Could you check a few things on this model? Use its own coordinates, in mm. Face numbers are marked on the shaded views. Give positions to 0.01 mm unless a question says otherwise; leave off trailing zeros. Write each loop counter-clockwise with the first axis right and the second up, starting at its lowest first coordinate (ties: lowest second). Pieces come first, ordered by that corner, then holes. Notation, with made-up numbers: (38.5, 61.25) - (83.5, 61.25) arc R17 ccw to (83.5, 78.25) - close; hole circle Ø6 at (53.25, -20). An arc over 180 degrees is marked (long way). Write item = value, one per line.
from build123d import *

# Parameters (mm, degrees)
SKETCH1_R           = 30
SKETCH1_R_2         = 5
BOSS_EXTRUDE1_DEPTH = 15
FILLET1_R           = 15


with BuildPart() as part:
    # Sketch1 → Boss-Extrude1 (new, symmetric)
    with BuildSketch(Plane(origin=(0, 0, 0), x_dir=(1, 0, 0), z_dir=(0, 1, 0))):
        with BuildLine():
            Line((13.821869985, 37.536061462), (7.39103626, 53.061467459))
            ThreePointArc((7.39103626, 53.061467459), (0, 58), (-7.39103626, 53.061467459))
            Line((-7.39103626, 53.061467459), (-13.821869985, 37.536061462))
            ThreePointArc((-13.821869985, 37.536061462), (-28.284271247, 28.284271247), (-37.536061462, 13.821869985))
            Line((-37.536061462, 13.821869985), (-53.061467459, 7.39103626))
            ThreePointArc((-53.061467459, 7.39103626), (-58, 0), (-53.061467459, -7.39103626))
            Line((-53.061467459, -7.39103626), (-37.536061462, -13.821869985))
            ThreePointArc((-37.536061462, -13.821869985), (-28.284271247, -28.284271247), (-13.821869985, -37.536061462))
            Line((-13.821869985, -37.536061462), (-7.39103626, -53.061467459))
            ThreePointArc((-7.39103626, -53.061467459), (0, -58), (7.39103626, -53.061467459))
            Line((7.39103626, -53.061467459), (13.821869985, -37.536061462))
            ThreePointArc((13.821869985, -37.536061462), (28.284271247, -28.284271247), (37.536061462, -13.821869985))
            Line((37.536061462, -13.821869985), (53.061467459, -7.39103626))
            ThreePointArc((53.061467459, -7.39103626), (58, 0), (53.061467459, 7.39103626))
            Line((53.061467459, 7.39103626), (37.536061462, 13.821869985))
            ThreePointArc((37.536061462, 13.821869985), (28.284271247, 28.284271247), (13.821869985, 37.536061462))
        make_face()
        with Locations(Location((0, 0, 0), (0, 0, 270))):
            Circle(SKETCH1_R, mode=Mode.SUBTRACT)
        with Locations(Location((0, 50, 0), (0, 0, 270))):
            Circle(SKETCH1_R_2, mode=Mode.SUBTRACT)
        with Locations(Location((-50, 0, 0), (0, 0, 270))):
            Circle(SKETCH1_R_2, mode=Mode.SUBTRACT)
        with Locations(Location((50, 0, 0), (0, 0, 270))):
            Circle(SKETCH1_R_2, mode=Mode.SUBTRACT)
        with Locations(Location((0, -50, 0), (0, 0, 270))):
            Circle(SKETCH1_R_2, mode=Mode.SUBTRACT)
    extrude(amount=BOSS_EXTRUDE1_DEPTH, both=True)

    # Fillet1
    fillet1_edges = [part.edges().sort_by_distance(p)[0] for p in [
        (-37.536061462, 0, -13.821869985),
        (-13.821869985, 0, -37.536061462),
        (13.821869985, 0, -37.536061462),
        (37.536061462, 0, -13.821869985),
        (37.536061462, 0, 13.821869985),
        (13.821869985, 0, 37.536061462),
        (-13.821869985, 0, 37.536061462),
        (-37.536061462, 0, 13.821869985),
    ]]
    fillet(fillet1_edges, radius=FILLET1_R)


solid = part.part
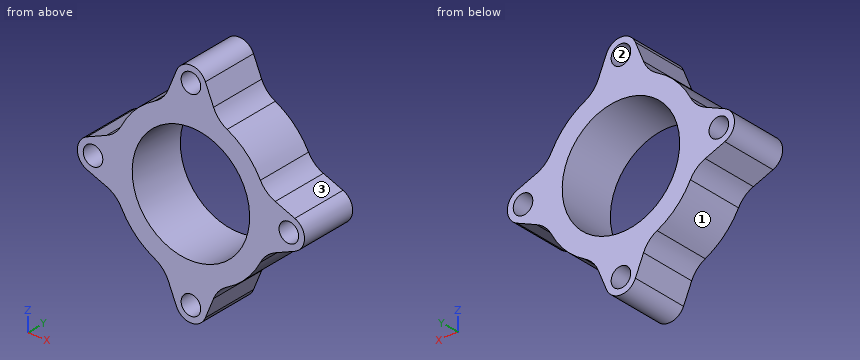
1. If we section it at C-C, the plane y = 2.25: Count the separate pieces of the cut face and the enclosed holes in it, and give its area (3 significant figures).
Filled sheet:
separate_pieces = 1
enclosed_holes = 5
area = 3,260 mm2
2. I need wall thicknesses on line 1 (X direction, y = -7.25, z = 0); line 2 (X direction, y = 4.25, z = -1.5); line 3 (Z direction, x = 9.5, y = 7.25). Which ranges of each line are inside material? Lowest first, please.
Filled sheet:
line_1 = -58 to -55, -45 to -30, 30 to 45, 55 to 58
line_2 = -57.86 to -54.77, -45.23 to -29.96, 29.96 to 45.23, 54.77 to 57.86
line_3 = -47.97 to -28.46, 28.46 to 47.97
3. If we section it at A-A, the plane x = 0: Please give me the cut outline in (y, z).
Filled sheet:
outline = (-15, -58) - (15, -58) - (15, -55) - (-15, -55) - close; (-15, -45) - (15, -45) - (15, -30) - (-15, -30) - close; (-15, 30) - (15, 30) - (15, 45) - (-15, 45) - close; (-15, 55) - (15, 55) - (15, 58) - (-15, 58) - close
4. If we section it at B-B, the plane z = 0: Please give me the cut outline in (x, y), and give its area (3 significant figures).
Filled sheet:
outline = (-58, -15) - (-55, -15) - (-55, 15) - (-58, 15) - close; (-45, -15) - (-30, -15) - (-30, 15) - (-45, 15) - close; (30, -15) - (45, -15) - (45, 15) - (30, 15) - close; (55, -15) - (58, -15) - (58, 15) - (55, 15) - close
area = 1,080 mm2
5. Thinking about a two-plate mould opening in X: for the marked faces 1, 2 and 3, which applies, pulls with the +X half, pulls with the -X half, needs draft (parallel to the pull), parting line crosses it, or undercut?
Filled sheet:
face_1 = pulls with the -X half
face_2 = undercut
face_3 = pulls with the +X half
6. For pin 1 (1 mm diameter, centred on y = -5.5, z = -32, fed in from -X); pin 2 (10 mm diameter, centred on x = 44, y = 0.5, fed in from -Z); pin 3 (4 mm diameter, centred on y = -4.5, z = -44, fed in from +X); pin 4 (5 mm diameter, centred on x = -36, z = 23.5, fed in from -Y) (3 decimals), each with a flat end and sliding along its axis, tell me the tip position at first contact or that it passes through.
Filled sheet:
pin_1 = -24.65
pin_2 = -14.03
pin_3 = 12.02
pin_4 = through
7. If we section it at D-D, the plane x = -22: Please give me the cut outline in (y, z), and give its area (3 significant figures).
Filled sheet:
outline = (-15, -33.41) - (15, -33.41) - (15, -20.4) - (-15, -20.4) - close; (-15, 20.4) - (15, 20.4) - (15, 33.41) - (-15, 33.41) - close
area = 781 mm2
